from build123d import *

# Parameters (mm, degrees)
F0_W     = 25.4
F0_H     = 76.2
F1_DEPTH = 2.54
F2_W     = 25.4
F2_H     = 12.7
F3_DEPTH = 19.05
F5_D     = 2.7051
F7_DEPTH = 21.591
F8_R     = 8.89


with BuildPart() as f1:
    # F0 (on Front) → F1 (new body)
    with BuildSketch(Plane.XZ):
        with Locations((12.7, 38.1)):
            Rectangle(F0_W, F0_H)
    extrude(amount=F1_DEPTH)

    # F2 (on face) → F3 (join)
    with BuildSketch(Plane(origin=(0, 0, 0), x_dir=(-1, 0, 0), z_dir=(0, 1, 0))):
        with Locations((-12.7, 69.85)):
            Rectangle(F2_W, F2_H)
    extrude(amount=F3_DEPTH)

    # F5 (through all)
    with Locations(Plane(origin=(0, 0, 63.5), x_dir=(1, 0, 0), z_dir=(0, 0, -1))):
        with Locations((12.7, -8.255)):
            Hole(F5_D / 2)

    # F6 (on face) → F7 (cut, through all)
    with BuildSketch(Plane.XZ.offset(2.54)):
        with BuildLine():
            ThreePointArc((15.24, 38.735), (12.7, 41.275), (10.16, 38.735))
            Line((10.16, 38.735), (10.16, 13.335))
            ThreePointArc((10.16, 13.335), (12.7, 10.795), (15.24, 13.335))
            Line((15.24, 13.335), (15.24, 38.735))
        make_face()
    extrude(amount=-F7_DEPTH, mode=Mode.SUBTRACT)

    # F8
    f8_edges = [f1.edges().sort_by_distance(p)[0] for p in [
        (0, -1.27, 0),
        (25.4, -1.27, 0),
    ]]
    fillet(f8_edges, radius=F8_R)


solid = f1.part
Design review of the part built by this model. Coordinates are the model's own, in mm. A direction names the side the tool comes from. Round coordinates to 2 decimals unless told otherwise and drop trailing zeros. Write each loop counter-clockwise with the first axis right and the second up, starting at its lowest first coordinate (ties: lowest second). Pieces come first, ordered by that corner, then holes. Notation, with made-up numbers: M 51.25,77.5 L 61.25,77.5 A26 ccw 61.25,106.5 Z; hole C -31.5,32 d7. An arc over 180 degrees is marked long. One line per item, written item: value. Start each with the question number.
1. Clearance check with flat-ended pins moving along their axes: P1, Ø7.5, axis at x = 9, z = 27, coming from the +Y side; P2, Ø2.5, axis at x = 12.7, y = 8.255, coming from the -Z side. State where each tip first meets the part, or that it passes through.
2. Take a section at B-B on z = 27.5. State the section outline as (x, y) points.
3. To check wall thickness, follow probe 1 along Y at (x, z) = (12.7, 67.5); probe 2 along Y at (x, z) = (7.75, 21); probe 3 along Z at (x, y) = (17.75, 10.5). State the ranges of each line that lie inside material, in increasing order. Write a range as from..to.
4. Draft analysis for pull direction Y (two halves, no side actions). For faces 4 (the face through (15.24, -1, 26)), 5 (the face through (10, -2.54, 39)), 6 (the face through (13, 19.05, 70)), 7 (the face through (12.993, 9.575, 69.939)), state which applies: pulls with the +Y half, pulls with the -Y half, needs draft (parallel to the pull), parting line crosses it, or undercut.
5. Take a section at A-A on x = 12.7. State the section outline as (y, z) points (3 decimals), then the cut area to 3 significant figures.
6. For faces 1 (the face through (0, -1, 60)), 2 (the face through (13, 12, 63.5)), 3 (the face through (10.16, -1, 26)), list the 3-axis set-ups (+Z, -Z, +X, -X, +Y, -Y) from which the entire face can be reached by the end or side of a thin tool; tool diameter is ignored.
7. Take a section at C-C on y = 10.5. State the section outline as (x, z) points, then the cut area to 3 significant figures.
8. Take a section at D-D on x = 19.5. State the section outline as (y, z) points, then the cut area to 3 significant figures.
Computed:
1. P1: stops at y = 0
1. P2: passes through
2. outline: M 0,-2.54 L 10.16,-2.54 L 10.16,0 L 0,0 Z; M 15.24,-2.54 L 25.4,-2.54 L 25.4,0 L 15.24,0 Z
3. probe 1: y = -2.54..6.9, 9.61..19.05
3. probe 2: y = -2.54..0
3. probe 3: z = 63.5..76.2
4. face 4: needs draft
4. face 5: pulls with the -Y half
4. face 6: pulls with the +Y half
4. face 7: undercut
5. outline: M -2.54,0 L 0,0 L 0,10.795 L -2.54,10.795 Z; M -2.54,41.275 L 0,41.275 L 0,63.5 L 6.902,63.5 L 6.902,76.2 L -2.54,76.2 Z; M 9.608,63.5 L 19.05,63.5 L 19.05,76.2 L 9.608,76.2 Z
5. area: 324 mm²
6. face 1: +Z, -Z, -X, +Y, -Y
6. face 2: -Z, +X, -X, +Y
6. face 3: +Y, -Y
7. outline: M 0,63.5 L 25.4,63.5 L 25.4,76.2 L 0,76.2 Z
7. area: 323 mm²
8. outline: M -2.54,0.52 L 0,0.52 L 0,63.5 L 19.05,63.5 L 19.05,76.2 L -2.54,76.2 Z
8. area: 434 mm²
